Design review of the part shown in the three views and the two pictorial views. Dimensions are in mm from the part's minimum x, y and z. A direction names the side the tool comes from. Round coordinates to 2 decimals unless told otherwise and drop trailing zeros. Write each loop counter-clockwise with the first axis right and the second up, starting at its lowest first coordinate (ties: lowest second). Pieces come first, ordered by that corner, then holes. Notation, with made-up numbers: (56, 54.25) -> (89, 54.25) arc R21 cw to (89, 69.25) -> close; hole circle Ø1 at (31.5, 5). An arc over 180 degrees is marked (long way). Return JSON: item names as keys, results as strings. Group by question number.
1. Clearance check with flat-ended pins moving along their axes: P1, Ø1.5, axis at x = 9.5, z = 5, coming from the +Y side; P2, Ø0.8, axis at x = 6.5, y = 4.5, coming from the +Z side; P3, Ø2, axis at x = 8, y = 3, coming from the +Z side; P4, Ø2.5, axis at y = 4.25, z = 6, coming from the +X side (3 decimals). State where each tip first meets the part, or that it passes through.
2. Mouldability with a two-part tool opening along Y and no side actions: class the marked faces 1, 2 and 3 as pulls with the +Y half, pulls with the -Y half, needs draft (parallel to the pull), parting line crosses it, or undercut.
3. Take a section at C-C, the plane z = 6. Write out the cut boundary in (x, y) (3 decimals).
4. Take a section at A-A, the plane z = 8.5. Write out the cut boundary in (x, y) (3 decimals), then the cut area to 3 significant figures.
5. Take a section at D-D, the plane x = 6.25. Write out the cut boundary in (y, z) (3 decimals).
6. Take a section at B-B, the plane y = 4.25. Write out the cut boundary in (x, z) (3 decimals), then the cut area to 4 significant figures.
7. Tool access review of the marked faces 4, 5, 6, 7 and 8: name each direction out of +Z, -Z, +X, -X, +Y, -Y from which nothing blocks a thin tool from reaching the whole face with its end or side.
8. For line 1 along Z through (x, y) = (1.3, 4.25); line 2 along Y through (x, z) = (6.25, 6) (3 decimals); line 3 along Z through (x, y) = (7.25, 7), list the stretches that pass through material, from the lowest coordinate up. Write a range as from..to.
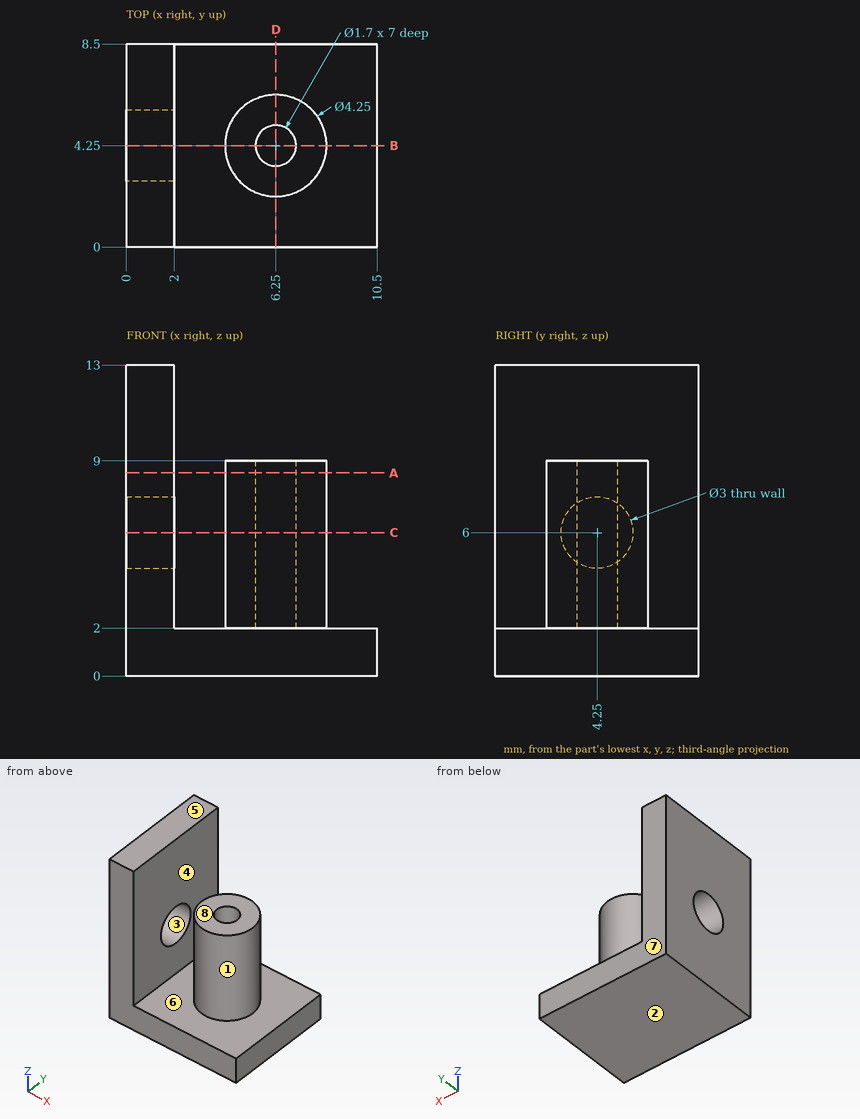
Output:
{
 "1": {"P1": "passes through", "P2": "stops at z = 2", "P3": "stops at z = 9", "P4": "stops at x = 8.375"},
 "2": {"face 1": "parting line crosses it", "face 2": "needs draft", "face 3": "undercut"},
 "3": {"outline": "(0, 0) -> (2, 0) -> (2, 2.75) -> (0, 2.75) -> close; (0, 5.75) -> (2, 5.75) -> (2, 8.5) -> (0, 8.5) -> close; circle Ø4.25 at (6.25, 4.25); hole circle Ø1.7 at (6.25, 4.25)"},
 "4": {"outline": "(0, 0) -> (2, 0) -> (2, 8.5) -> (0, 8.5) -> close; circle Ø4.25 at (6.25, 4.25); hole circle Ø1.7 at (6.25, 4.25)", "area": "28.9 mm^2"},
 "5": {"outline": "(0, 0) -> (8.5, 0) -> (8.5, 2) -> (6.375, 2) -> (6.375, 9) -> (5.1, 9) -> (5.1, 2) -> (3.4, 2) -> (3.4, 9) -> (2.125, 9) -> (2.125, 2) -> (0, 2) -> close"},
 "6": {"outline": "(0, 0) -> (10.5, 0) -> (10.5, 2) -> (8.375, 2) -> (8.375, 9) -> (7.1, 9) -> (7.1, 2) -> (5.4, 2) -> (5.4, 9) -> (4.125, 9) -> (4.125, 2) -> (2, 2) -> (2, 4.5) -> (0, 4.5) -> close; (0, 7.5) -> (2, 7.5) -> (2, 13) -> (0, 13) -> close", "area": "54.85 mm^2"},
 "7": {"face 4": "+Z, +Y, -Y", "face 5": "+Z, +X, -X, +Y, -Y", "face 6": "+Z", "face 7": "+Z, -Z, +X, -X, +Y", "face 8": "+Z, +X, +Y, -Y"},
 "8": {"line 1": "z = 0..4.5, 7.5..13", "line 2": "y = 2.125..3.4, 5.1..6.375", "line 3": "z = 0..2"}
}
